Could you check a few things on this model? Use its own coordinates, in mm. Face numbers are marked on the shaded views. A direction names the side the tool comes from. Round coordinates to 2 decimals unless told otherwise and drop trailing zeros. Order: outer loops, then holes, each group sorted by start corner. A loop starts at its lowest first (then second) coordinate and runs counter-clockwise, first axis right, second up. Notation, with made-up numbers: M 39,88.25 L 58,88.25 A27 ccw 58,116.25 Z; hole C -36,30 d8. An arc over 180 degrees is marked long. Write each question's results on one line, items separated by ' | '. Start each with the question number.
1. I'm going to push a flat-ended pin straight in: pin 1 (1 mm diameter, centred on x = 1.5, z = -9, fed in from +Y). Where does the tip first touch, or does it pass through?
2. Suppose I cut it at B-B on z = -10. Write out the boundary of the cut face in (x, y), and give its area (3 significant figures).
3. Suppose I cut it at D-D on y = 4. Write out the boundary of the cut face in (x, z).
4. Please list where this line runs through material, in increasing order: L1, parallel to X at y = 6, z = -4.
5. For the marked faces 4 and 5, which set-ups out of +Z, -Z, +X, -X, +Y, -Y let a thin tool reach every point of the face, with its end or its side?
6. Suppose I cut it at C-C on x = 1. Write out the boundary of the cut face in (y, z).
7. Suppose I cut it at A-A on y = 15. Write out the boundary of the cut face in (x, z).
8. We'd pull the mould along Y, two halves only. Please class the marked faces 1, 2 and 3: released by +Y, released by -Y, zero draft, split by the parting line, or undercut.
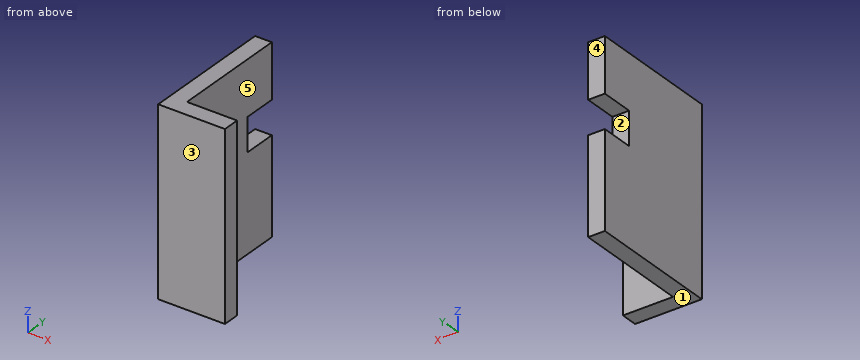
Autodesk Inventor part; units mm, degrees
ref_plane "YZ Plane" through (0, 0, 0) normal (1, 0, 0) x (0, 1, 0)
ref_plane "XZ Plane" through (0, 0, 0) normal (0, 1, 0) x (-1, 0, 0)
ref_plane "XY Plane" through (0, 0, 0) normal (0, 0, 1) x (1, 0, 0)
sketch "Sketch1" plane through (0, 0, 0) normal (0, 0, 1) x (1, 0, 0)
  line L0 (0, 0) -> (2, 0)
  line L1 (2, 0) -> (2, 16)
  line L2 (2, 16) -> (0, 16)
  line L3 (0, 16) -> (0, 0)
  line L4 (2, 2) -> (8, 2)
  line L5 (8, 2) -> (8, 0)
  line L6 (8, 0) -> (2, 0)
  line L7 (2, 0) -> (2, 2)
  dimension "d0" = 2
  dimension "d1" = 16
  dimension "d2" = 6
extrude "Extrusion1" add sketch "Sketch1" against normal blind 22
sketch "Sketch2" plane through (2, 2, 0) normal (1, 0, 0) x (0, 0, -1)
  line L0 (10.5, 14) -> (6.5, 14)
  line L1 (6.5, 14) -> (6.5, 10)
  line L2 (6.5, 10) -> (10.5, 10)
  line L3 (10.5, 10) -> (10.5, 14)
  point P0 (0, -2)
  dimension "d5" = 4
  dimension "d6" = 4
extrude "Extrusion2" cut sketch "Sketch2" against normal blind 10
properties part number "housing_mate_v04"
Filled sheet:
1) pin 1: stops at y = 12
2) outline: M 0,0 L 8,0 L 8,2 L 2,2 L 2,12 L 0,12 Z | area: 36.0 mm^2
3) outline: M 0,-22 L 2,-22 L 2,0 L 0,0 Z
4) L1: x = 0 to 2
5) face 4: +Z, -Z, +X, -X, +Y | face 5: +Z, -Z, +X, +Y
6) outline: M 0,-22 L 16,-22 L 16,-10.5 L 12,-10.5 L 12,-6.5 L 16,-6.5 L 16,0 L 0,0 Z
7) outline: M 0,-22 L 2,-22 L 2,-10.5 L 0,-10.5 Z; M 0,-6.5 L 2,-6.5 L 2,0 L 0,0 Z
8) face 1: zero draft | face 2: released by +Y | face 3: released by -Y
